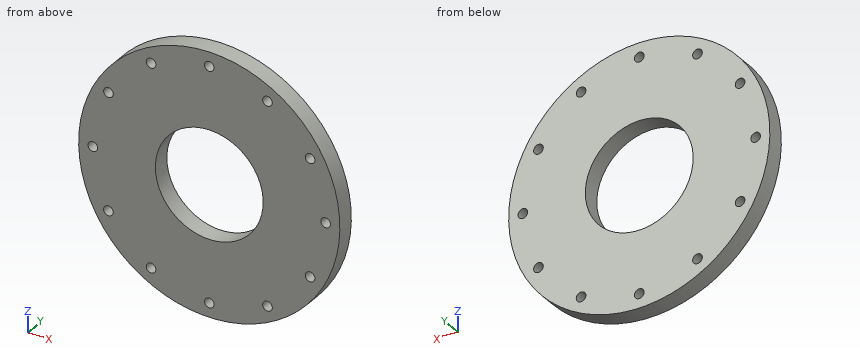
```python
from build123d import *

# Parameters (mm, degrees)
SKETCH2_W            = 27
SKETCH2_H            = 6.35
M3_CLEARANCE_HOLE1_D = 3.4
CIRPATTERN1_COUNT    = 12


with BuildPart() as part:
    # Sketch2 → Revolve1 (revolve)
    with BuildSketch(Plane(origin=(0, 0, 0), x_dir=(0, 0, -1), z_dir=(1, 0, 0))):
        with Locations((-32.5, 3.175)):
            Rectangle(SKETCH2_W, SKETCH2_H)
    revolve(axis=Axis((0, 0, 0), (0, 1, 0)))

    # M3 Clearance Hole1 (through all)
    with Locations(Plane(origin=(0, 6.35, 0), x_dir=(1, 0, 0), z_dir=(0, 1, 0))):
        with Locations((0, 41)):
            m3_clearance_hole1 = Hole(M3_CLEARANCE_HOLE1_D / 2)

    # CirPattern1: M3 Clearance Hole1 ×12 about axis
    cirpattern1_axis = Axis((0, 0, 0), (0, 1, 0))
    for i in range(1, CIRPATTERN1_COUNT):
        add(m3_clearance_hole1.rotate(cirpattern1_axis, i * 360 / CIRPATTERN1_COUNT), mode=Mode.SUBTRACT)


solid = part.part
```
Read the model definition and answer for the solid it produces. Units are mm, in the model's axes. Round coordinates to 2 decimals unless told otherwise and drop trailing zeros. Write each loop counter-clockwise with the first axis right and the second up, starting at its lowest first coordinate (ties: lowest second). Pieces come first, ordered by that corner, then holes. Notation, with made-up numbers: (36, -13) -> (95, -13) arc R28 cw to (95, 14) -> close; hole circle Ø8 at (60, 66.5). An arc over 180 degrees is marked (long way). Answer in a Markdown table with one row per item. Add a question column.
1) Given P1, Ø4, axis at x = 0, z = -41, coming from the -Y side; P2, Ø2.5, axis at x = 35.51, z = 20.5, coming from the -Y side, each flat-ended and moving along its own axis, determine where each tip first touches the part or whether it passes through.
2) Consider line 1 (X direction, y = 4.75, z = 0); line 2 (Z direction, x = -34, y = 3); line 3 (Z direction, x = 1, y = 4). Determine where each line is inside the solid, lowest interval first.
3) Find section B-B, the plane x = 13.5. Determine the outline of the cut face in (y, z), and give its area (3 significant figures).
4) Find section C-C, the plane z = 20.5. Determine the outline of the cut face in (x, y), and give its area (3 significant figures).
5) Find section A-A, the plane z = 5.5. Determine the outline of the cut face in (x, y), and give its area (3 significant figures).
6) Find section D-D, the plane y = 4.5. State how many separate pieces and enclosed holes the cut face has, and give its area (3 significant figures).
Findings below:
| question | item | result |
|---|---|---|
| 1 | P1 | y = 0 |
| 1 | P2 | through |
| 2 | line 1 | -46 to -42.7, -39.3 to -19, 19 to 39.3, 42.7 to 46 |
| 2 | line 2 | -30.98 to -21.29, -19.71 to 19.71, 21.29 to 30.98 |
| 2 | line 3 | -45.99 to -42.37, -39.63 to -18.97, 18.97 to 39.63, 42.37 to 45.99 |
| 3 | outline | (0, -43.97) -> (6.35, -43.97) -> (6.35, -13.37) -> (0, -13.37) -> close; (0, 13.37) -> (6.35, 13.37) -> (6.35, 43.97) -> (0, 43.97) -> close |
| 3 | area | 389 mm² |
| 4 | outline | (-41.18, 0) -> (-37.21, 0) -> (-37.21, 6.35) -> (-41.18, 6.35) -> close; (-33.81, 0) -> (33.81, 0) -> (33.81, 6.35) -> (-33.81, 6.35) -> close; (37.21, 0) -> (41.18, 0) -> (41.18, 6.35) -> (37.21, 6.35) -> close |
| 4 | area | 480 mm² |
| 5 | outline | (-45.67, 0) -> (-18.19, 0) -> (-18.19, 6.35) -> (-45.67, 6.35) -> close; (18.19, 0) -> (45.67, 0) -> (45.67, 6.35) -> (18.19, 6.35) -> close |
| 5 | area | 349 mm² |
| 6 | separate pieces | 1 |
| 6 | enclosed holes | 13 |
| 6 | area | 5,400 mm² |
